The model under review builds one solid part; all positions refer to its coordinate system, in mm. Face numbers are marked on the shaded views. Round coordinates to 2 decimals unless told otherwise and drop trailing zeros. Order: outer loops, then holes, each group sorted by start corner. A loop starts at its lowest first (then second) coordinate and runs counter-clockwise, first axis right, second up. Notation, with made-up numbers: (44, 84) -> (78, 84) arc R37 cw to (78, 123) -> close; hole circle Ø5 at (-14.5, 24). An arc over 180 degrees is marked (long way). Put each result on its own line as item: value. Start each with the question number.
from build123d import *

# Parameters (mm, degrees)
SKETCH_1_W          = 29
SKETCH_1_H          = 29
SKETCH_1_W_2        = 19
SKETCH_1_H_2        = 19
EXTRUDE_1_DEPTH     = 50
SKETCH_2_W          = 29
SKETCH_2_H          = 29
EXTRUDE_2_DEPTH     = 5
SKETCH_3_W          = 10
SKETCH_3_H          = 10
EXTRUDE_3_DEPTH     = 10
CUT_EXTRUDE_1_DEPTH = 10
SKETCH_7_W          = 130
SKETCH_7_H          = 190
EXTRUDE_4_DEPTH     = 3
CUT_EXTRUDE_2_DEPTH = 165.058536671
SKETCH_10_R         = 1.25
CUT_EXTRUDE_3_DEPTH = 149.400384885
CUT_EXTRUDE_9_DEPTH = 3
FILLET_1_R          = 2
FILLET_3_R          = 5


with BuildPart() as part:
    # 草图1 → 凸台-拉伸1 (new body)
    with BuildSketch(Plane.XY):
        Rectangle(SKETCH_1_W, SKETCH_1_H)
        Rectangle(SKETCH_1_W_2, SKETCH_1_H_2, mode=Mode.SUBTRACT)
    extrude(amount=EXTRUDE_1_DEPTH)

    # 草图2 → 凸台-拉伸2 (add)
    with BuildSketch(Plane.XY.offset(50)):
        Rectangle(SKETCH_2_W, SKETCH_2_H)
    extrude(amount=EXTRUDE_2_DEPTH)

    # 草图3 → 凸台-拉伸3 (add)
    with BuildSketch(Plane.XY.offset(55)):
        Rectangle(SKETCH_3_W, SKETCH_3_H)
    extrude(amount=EXTRUDE_3_DEPTH)

    # 草图4 → 切除-拉伸1 (cut)
    with BuildSketch(Plane(origin=(0, 5, 0), x_dir=(1, 0, 0), z_dir=(0, 1, 0))):
        Polygon((-5, -55), (5, -65), (-5, -65), align=None)
    extrude(amount=-CUT_EXTRUDE_1_DEPTH, mode=Mode.SUBTRACT)

    # 草图7 → 凸台-拉伸4 (add)
    with BuildSketch(Plane(origin=(-30, 0, 30), x_dir=(0.7071067811865475, 0, 0.7071067811865476), z_dir=(-0.7071067811865476, 0, 0.7071067811865475))):
        with Locations((47.497474683, 0)):
            Rectangle(SKETCH_7_W, SKETCH_7_H)
    extrude(amount=EXTRUDE_4_DEPTH)

    # 草图8 → 切除-拉伸2 (cut, through all)
    with BuildSketch(Plane.XZ.offset(14.5)):
        Polygon((-14.5, 55), (-14.5, 49.742640687), (-9.242640687, 55), align=None)
    extrude(amount=-CUT_EXTRUDE_2_DEPTH, mode=Mode.SUBTRACT)

    # 草图10 → 切除-拉伸3 (cut, through all)
    with BuildSketch(Plane(origin=(-32.121320344, 0, 32.121320344), x_dir=(0.7071067811865475, 0, 0.7071067811865476), z_dir=(-0.7071067811865476, 0, 0.7071067811865475))):
        with Locations((107.497474683, 90)):
            Circle(SKETCH_10_R)
        with Locations((-12.502525317, 90)):
            Circle(SKETCH_10_R)
        with Locations((-12.502525317, -91)):
            Circle(SKETCH_10_R)
        with Locations((107.497474683, -90)):
            Circle(SKETCH_10_R)
    extrude(amount=-CUT_EXTRUDE_3_DEPTH, mode=Mode.SUBTRACT)

    # 草图11 → 切除-拉伸9 (cut)
    with BuildSketch(Plane(origin=(-32.121320344, 0, 32.121320344), x_dir=(0.7071067811865475, 0, 0.7071067811865476), z_dir=(-0.7071067811865476, 0, 0.7071067811865475))):
        Polygon((-0.25988463, -82), (95.254833996, -82), (91.254833996, -78), (3.74011537, -78), align=None)
        Polygon((99.497474683, -77.757359313), (99.497474683, 77.757359313), (95.497474683, 73.757359313), (95.497474683, -73.757359313), align=None)
        Polygon((-0.502525317, 73.757359313), (-4.502525317, 77.757359313), (-4.502525317, -77.757359313), (-0.502525317, -73.757359313), align=None)
        Polygon((91.254833996, 78), (95.254833996, 82), (-0.25988463, 82), (3.74011537, 78), align=None)
    extrude(amount=-CUT_EXTRUDE_9_DEPTH, mode=Mode.SUBTRACT)

    # 圆角1
    fillet_1_edges = [part.edges().sort_by_distance(p)[0] for p in [
        (5, 0, 55),
        (0, 5, 55),
        (5, 5, 60),
        (5, -5, 60),
        (0, -5, 55),
        (4.75, -14.5, 55),
        (-14.5, -14.5, 22.75),
        (-14.5, 14.5, 22.75),
        (4.75, 14.5, 55),
        (-28.415999231, 78, 33.705321112),
        (-31.244426356, 82, 30.876893988),
        (36.294678888, 82, 98.415999231),
        (33.466251763, 78, 95.587572106),
        (-31.415999231, -73.757359313, 30.705321112),
        (-34.244426356, -77.757359313, 27.876893988),
        (-34.244426356, 77.757359313, 27.876893988),
        (-31.415999231, 73.757359313, 30.705321112),
        (36.466251763, 73.757359313, 98.587572106),
        (39.294678888, 77.757359313, 101.415999231),
        (39.294678888, -77.757359313, 101.415999231),
        (36.466251763, -73.757359313, 98.587572106),
        (33.466251763, -78, 95.587572106),
        (-31.244426356, -82, 30.876893988),
        (-28.415999231, -78, 33.705321112),
        (36.294678888, -82, 98.415999231),
    ]]
    fillet(fillet_1_edges, radius=FILLET_1_R - 0.0001)  # a hair under: the kernel refuses the full size

    # 圆角3
    fillet_3_edges = [part.edges().sort_by_distance(p)[0] for p in [
        (-43.436814511, 95, 18.684505832),
        (-43.436814511, -95, 18.684505832),
        (48.487067043, -95, 110.608387387),
        (48.487067043, 95, 110.608387387),
    ]]
    fillet(fillet_3_edges, radius=FILLET_3_R)


solid = part.part
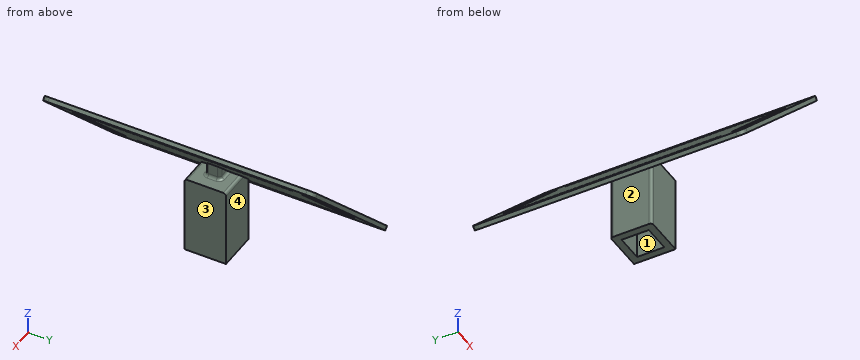
Q1. Wall thickness on probe 1 along Y at (x, z) = (-9, 48); probe 2 along X at (y, z) = (-1.5, 23.5); probe 3 along Y at (x, z) = (1.5, 53.5): over which ranges is each line inside the solid? List them lowest first. Write a range as [from, to].
Q2. Take a section at A-A on z = 42. Give the boundary of the cut face in (x, y).
Q3. Take a section at C-C on z = 9.5. Give the boundary of the cut face in (x, y).
Q4. Take a section at B-B on y = 46.5. Give the boundary of the cut face in (x, z).
Q5. Draft analysis for pull direction X (two halves, no side actions). For the marked faces 1, 2, 3 and 4, state which applies: +X half, -X half, draft (parallel to the pull), parting line (faces both ways), or undercut.
Q6. Take a section at D-D on x = 0. Give the boundary of the cut face in (y, z).
Q7. Clearance check with flat-ended pins moving along their axes: pin 1 Ø1 at (x, y) = (32, 6) entering from +Z; pin 2 Ø5.5 at (x, z) = (-2.5, 22) entering from -Y; pin 3 Ø1 at (x, z) = (-14.5, 34) entering from +Y. State where each tip first meets the part, or that it passes through.
Calculated:
1. probe 1: y = [-14.5, -9.5], [9.5, 14.5]
1. probe 2: x = [-40.74, -36.5], [-14.5, -9.5], [9.5, 14.5]
1. probe 3: y = [-14.44, 14.44]
2. outline: (-22.24, -95) -> (-18, -95) -> (-18, -82) -> (-22.24, -82) -> close; (-22.24, -78) -> (-18, -78) -> (-18, 78) -> (-22.24, 78) -> close; (-22.24, 82) -> (-18, 82) -> (-18, 95) -> (-22.24, 95) -> close; (-14.5, -12.5) arc R2 ccw to (-12.5, -14.5) -> (14.5, -14.5) -> (14.5, 14.5) -> (-12.5, 14.5) arc R2 ccw to (-14.5, 12.5) -> close; hole (-9.5, -9.5) -> (9.5, -9.5) -> (9.5, 9.5) -> (-9.5, 9.5) -> close
3. outline: (-14.5, -12.5) arc R2 ccw to (-12.5, -14.5) -> (14.5, -14.5) -> (14.5, 14.5) -> (-12.5, 14.5) arc R2 ccw to (-14.5, 12.5) -> close; hole (-9.5, -9.5) -> (9.5, -9.5) -> (9.5, 9.5) -> (-9.5, 9.5) -> close
4. outline: (-44.5, 19.75) -> (-42.38, 17.62) -> (-33.18, 26.82) -> (-35.31, 28.94) -> close; (-32.48, 31.77) -> (-30.36, 29.64) -> (37.53, 97.53) -> (35.41, 99.65) -> close; (38.23, 102.48) -> (40.36, 100.36) -> (49.55, 109.55) -> (47.43, 111.67) -> close
5. face 1: undercut
5. face 2: undercut
5. face 3: +X half
5. face 4: draft
6. outline: (-95, 60) -> (-82, 60) -> (-82, 64.24) -> (-95, 64.24) -> close; (-78, 60) -> (-5, 60) -> (-5, 57) arc R2 cw to (-7, 55) -> (-12.5, 55) arc R2 ccw to (-14.5, 53) -> (-14.5, 0) -> (-9.5, 0) -> (-9.5, 50) -> (9.5, 50) -> (9.5, 0) -> (14.5, 0) -> (14.5, 53) arc R2 ccw to (12.5, 55) -> (7, 55) arc R2 cw to (5, 57) -> (5, 60) -> (78, 60) -> (78, 64.24) -> (-78, 64.24) -> close; (82, 60) -> (95, 60) -> (95, 64.24) -> (82, 64.24) -> close
7. pin 1: stops at z = 96.74
7. pin 2: stops at y = -14.5
7. pin 3: stops at y = 13.82
